```python
from build123d import *

# Parameters (mm, degrees)
SKETCH1_R           = 1.5
SKETCH1_R_2         = 2.75
SKETCH1_R_3         = 5
BOSS_EXTRUDE1_DEPTH = 3


with BuildPart() as part:
    # Sketch1 → Boss-Extrude1 (new body)
    with BuildSketch(Plane(origin=(0, 0, 0), x_dir=(1, 0, 0), z_dir=(0, 1, 0))):
        with BuildLine():
            Line((-15, 21.693547428), (-15, 38.108016468))
            ThreePointArc((-15, 38.108016468), (-14.121320344, 40.229336812), (-12, 41.108016468))
            Line((-12, 41.108016468), (12, 41.108016468))
            ThreePointArc((12, 41.108016468), (14.121320344, 40.229336812), (15, 38.108016468))
            Line((15, 38.108016468), (15, 21.693547428))
            ThreePointArc((15, 21.693547428), (15.631737063, 18.195598093), (17.447129909, 15.139605607))
            ThreePointArc((17.447129909, 15.139605607), (23.1, 0), (17.447129909, -15.139605607))
            ThreePointArc((17.447129909, -15.139605607), (15.631737063, -18.195598093), (15, -21.693547428))
            Line((15, -21.693547428), (15, -38.108016468))
            ThreePointArc((15, -38.108016468), (14.121320344, -40.229336812), (12, -41.108016468))
            Line((12, -41.108016468), (-12, -41.108016468))
            ThreePointArc((-12, -41.108016468), (-14.121320344, -40.229336812), (-15, -38.108016468))
            Line((-15, -38.108016468), (-15, -21.693547428))
            ThreePointArc((-15, -21.693547428), (-15.631737063, -18.195598093), (-17.447129909, -15.139605607))
            ThreePointArc((-17.447129909, -15.139605607), (-23.1, 0), (-17.447129909, 15.139605607))
            ThreePointArc((-17.447129909, 15.139605607), (-15.631737063, 18.195598093), (-15, 21.693547428))
        make_face()
        with Locations(Location((-8.838834765, 8.838834765, 0), (0, 0, 270))):
            Circle(SKETCH1_R, mode=Mode.SUBTRACT)
        with Locations(Location((8.838834765, -8.838834765, 0), (0, 0, 90))):
            Circle(SKETCH1_R, mode=Mode.SUBTRACT)
        with Locations(Location((6.717514421, 6.717514421, 0), (0, 0, 270))):
            Circle(SKETCH1_R_2, mode=Mode.SUBTRACT)
        with Locations(Location((-6.717514421, -6.717514421, 0), (0, 0, 90))):
            Circle(SKETCH1_R_2, mode=Mode.SUBTRACT)
        with Locations(Location((0, 0, 0), (0, 0, 270))):
            Circle(SKETCH1_R_3, mode=Mode.SUBTRACT)
        with Locations(Location((-8.838834765, 33.462792438, 0), (0, 0, 270))):
            Circle(SKETCH1_R, mode=Mode.SUBTRACT)
        with Locations(Location((8.838834765, 33.462792438, 0), (0, 0, 90))):
            Circle(SKETCH1_R, mode=Mode.SUBTRACT)
        with Locations(Location((8.838834765, -33.462792438, 0), (0, 0, 270))):
            Circle(SKETCH1_R, mode=Mode.SUBTRACT)
        with Locations(Location((-8.838834765, -33.462792438, 0), (0, 0, 90))):
            Circle(SKETCH1_R, mode=Mode.SUBTRACT)
    extrude(amount=BOSS_EXTRUDE1_DEPTH)


solid = part.part
```
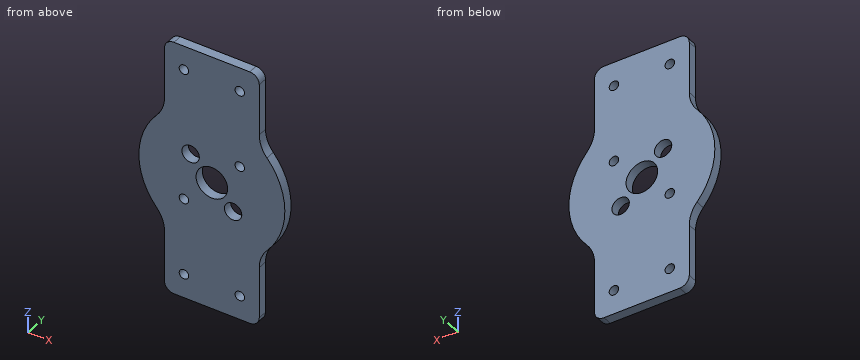
Can you work these out from the model? Positions are in its coordinate system, mm. Coordinates: 2 decimals unless noted, no trailing zeros. Loops run counter-clockwise (first coordinate to the right, second up) from the corner with the lowest first, then second, coordinate; pieces in that order, holes last.
Item 1: Please list where these lines run through material, in increasing order: L1, parallel to Z at x = 7, y = 0.45; L2, parallel to Z at x = -9, y = 2.7; L3, parallel to X at y = 0.7, z = 8.
Answers below:
L1: z = -41.11 to -9.45, -3.98 to 41.11
L2: z = -41.11 to -34.95, -31.97 to -10.33, -7.35 to 5.18, 8.25 to 31.97, 34.95 to 41.11
L3: x = -21.67 to -9.15, -4.28 to 7.6, 10.08 to 21.67
Item 2: Suppose I cut it at A-A (x = 3). Please give me the cut outline in (y, z), then the cut area to 3 significant figures.
Answers below:
outline: (0, -41.11) - (3, -41.11) - (3, -4) - (0, -4) - close; (0, 4) - (3, 4) - (3, 41.11) - (0, 41.11) - close
area: 223 mm2
Item 3: I'm going to push flat-ended pins straight in: pin 1 (2 mm diameter, centred on x = 0.5, z = -7.5, fed in from -Y); pin 2 (1.8 mm diameter, centred on x = -8.84, z = 33.46, fed in from -Y); pin 3 (1.5 mm diameter, centred on y = 2, z = -28.5, fed in from -X). Where does each tip first touch, or does it pass through?
Answers below:
pin 1: stops at y = 0
pin 2: passes through
pin 3: stops at x = -15
Item 4: Suppose I cut it at B-B (z = 0). Please give me the cut outline in (x, y).
Answers below:
outline: (-23.1, 0) - (-5, 0) - (-5, 3) - (-23.1, 3) - close; (5, 0) - (23.1, 0) - (23.1, 3) - (5, 3) - close
Item 5: Suppose I cut it at C-C (y = 2.35). State how many separate pieces and enclosed holes the cut face has, then the cut area to 3 significant figures.
Answers below:
separate pieces: 1
enclosed holes: 9
area: 2,690 mm2
